Build history of the part. All positions in model axes, mm. Face numbers are marked on the shaded views. Give positions to 0.01 mm unless a question says otherwise; leave off trailing zeros. Order: outer loops, then holes, each group sorted by start corner. A loop starts at its lowest first (then second) coordinate and runs counter-clockwise, first axis right, second up. Notation, with made-up numbers: (15.5, 87.5) -> (62.5, 87.5) arc R23 ccw to (62.5, 96.5) -> close; hole circle Ø3 at (22, 37.5). An arc over 180 degrees is marked (long way). One line per item, written item: value. Start each with the question number.
(1) Saw through at B-B on z = 21.75. Give the cut face in (x, y), plus the area to 4 significant figures.
(2) Saw through at D-D on x = 0. Give the cut face in (y, z), plus the area to 3 significant figures.
(3) Two-plate mould, pull along Y, no slides. Class the marked faces 1, 2, 3 and 4: +Y half, -Y half, draft (parallel to the pull), parting line (faces both ways), or undercut.
(4) Probe line 1 (Y direction, x = 10, z = 2.75); line 2 (Z direction, x = 23, y = 1.25); line 3 (Y direction, x = -2, z = 23.75). List the from-to ranges inside material, lowest first.
(5) Saw through at C-C on y = 1. Give the cut face in (x, z), plus the area to 3 significant figures.
(6) Pin check, flat tips, straight feed: pin 1 (0.5 mm diameter, centred on y = 3.5, z = 9, fed in from -X); pin 2 (2 mm diameter, centred on x = 3, y = 0, fed in from +Z); pin 3 (4 mm diameter, centred on y = 0, z = 19.5, fed in from +X); pin 4 (0.7 mm diameter, centred on x = -26.5, y = -3.5, fed in from +Z). Stop position of each tip, or through.
(7) Saw through at A-A on x = 21.5. Give the cut face in (y, z), plus the area to 3 significant figures.
```python
from build123d import *

# Parameters (mm, degrees)
SKETCH1_W           = 90
SKETCH1_H           = 8
BOSS_EXTRUDE1_DEPTH = 12.6
SKETCH2_W           = 90
SKETCH2_H           = 6.8
CUT_EXTRUDE1_DEPTH  = 12
BOSS_EXTRUDE2_DEPTH = 0.6
CUT_EXTRUDE2_DEPTH  = 9
CUT_EXTRUDE4_DEPTH  = 0.6
CUT_EXTRUDE5_DEPTH  = 0.6
FILLET1_R           = 0.6


with BuildPart() as part:
    # Sketch1 → Boss-Extrude1 (new body)
    with BuildSketch(Plane.XY):
        Rectangle(SKETCH1_W, SKETCH1_H)
    extrude(amount=BOSS_EXTRUDE1_DEPTH)

    # Sketch2 → Cut-Extrude1 (cut)
    with BuildSketch(Plane.XY.offset(12.6)):
        Rectangle(SKETCH2_W, SKETCH2_H)
    extrude(amount=-CUT_EXTRUDE1_DEPTH, mode=Mode.SUBTRACT)

    # Sketch8 → Boss-Extrude2 (add)
    with BuildSketch(Plane.XZ.offset(4)):
        with BuildLine():
            Line((6.4, 25.4), (13.6, 15.8))
            ThreePointArc((13.6, 15.8), (16.422291236, 13.444582472), (20, 12.6))
            Line((20, 12.6), (-20, 12.6))
            ThreePointArc((-20, 12.6), (-16.422291236, 13.444582472), (-13.6, 15.8))
            Line((-13.6, 15.8), (-6.4, 25.4))
            ThreePointArc((-6.4, 25.4), (0, 28.6), (6.4, 25.4))
        make_face()
    extrude(amount=-BOSS_EXTRUDE2_DEPTH)

    # Sketch4 → Cut-Extrude2 (cut, through all)
    with BuildSketch(Plane(origin=(0, 4, 0), x_dir=(1, 0, 0), z_dir=(0, 1, 0))):
        with BuildLine():
            Line((-1.5, -3.1), (-1.5, -32.05439328))
            Line((-1.5, -32.05439328), (1.5, -32.05439328))
            Line((1.5, -32.05439328), (1.5, -3.1))
            ThreePointArc((1.5, -3.1), (0, -1.6), (-1.5, -3.1))
        make_face()
    extrude(amount=-CUT_EXTRUDE2_DEPTH, mode=Mode.SUBTRACT)

    # Sketch6 → Cut-Extrude4 (cut)
    with BuildSketch(Plane(origin=(0, 4, 0), x_dir=(1, 0, 0), z_dir=(0, 1, 0))):
        with BuildLine():
            Line((-42.5, -9.1), (-42.5, -7.1))
            Line((-42.5, -7.1), (-45, -7.1))
            Line((-45, -7.1), (-45, -12.6))
            Line((-45, -12.6), (-39, -12.6))
            ThreePointArc((-39, -12.6), (-41.474873734, -11.574873734), (-42.5, -9.1))
        make_face()
    cut_extrude4 = extrude(amount=-CUT_EXTRUDE4_DEPTH, mode=Mode.SUBTRACT)

    # Mirror1: Cut-Extrude4 across plane
    add(cut_extrude4.mirror(Plane(origin=(0, 0, 0), x_dir=(0, 0, 1), z_dir=(1, 0, 0))), mode=Mode.SUBTRACT)

    # Sketch7 → Cut-Extrude5 (cut)
    with BuildSketch(Plane(origin=(0, 4, 0), x_dir=(1, 0, 0), z_dir=(0, 1, 0))):
        with BuildLine():
            Line((-4.5, -4.6), (-4.5, -6.6))
            ThreePointArc((-4.5, -6.6), (-6, -8.1), (-7.5, -6.6))
            Line((-7.5, -6.6), (-7.5, -4.6))
            ThreePointArc((-7.5, -4.6), (-6, -3.1), (-4.5, -4.6))
        make_face()
    cut_extrude5 = extrude(amount=-CUT_EXTRUDE5_DEPTH, mode=Mode.SUBTRACT)

    # Mirror2: Cut-Extrude5 across plane
    add(cut_extrude5.mirror(Plane(origin=(0, 0, 0), x_dir=(0, 0, 1), z_dir=(1, 0, 0))), mode=Mode.SUBTRACT)

    # Fillet1
    fillet1_edges = [part.edges().sort_by_distance(p)[0] for p in [
        (45, -3.7, 12.6),
        (-45, -3.7, 12.6),
        (-1.5, -3.7, 28.458116823),
        (1.5, -3.7, 28.458116823),
        (1.5, 3.7, 12.6),
        (-1.5, 3.7, 12.6),
        (-45, 3.7, 7.1),
        (45, 3.7, 7.1),
    ]]
    fillet(fillet1_edges, radius=FILLET1_R)


solid = part.part
```
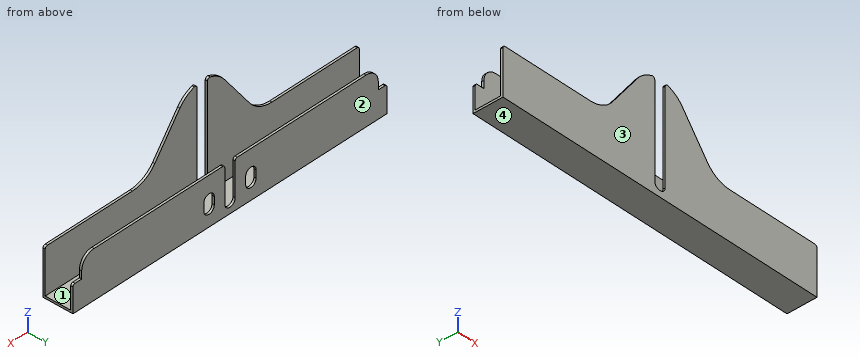
Results below:
1. outline: (-9.14, -4) -> (-1.5, -4) -> (-1.5, -3.4) -> (-9.14, -3.4) -> close; (1.5, -4) -> (9.14, -4) -> (9.14, -3.4) -> (1.5, -3.4) -> close
1. area: 9.165 mm²
2. outline: (-4, 0) -> (4, 0) -> (4, 1.6) -> (3.4, 1.6) -> (3.4, 0.6) -> (-3.4, 0.6) -> (-3.4, 1.6) -> (-4, 1.6) -> close
2. area: 6.00 mm²
3. face 1: undercut
3. face 2: +Y half
3. face 3: -Y half
3. face 4: draft
4. line 1: y = -4 to -3.4, 3.4 to 4
4. line 2: z = 0 to 0.6
4. line 3: y = -4 to -3.4
5. outline: (-45, 0) -> (45, 0) -> (45, 0.6) -> (-45, 0.6) -> close
5. area: 54.0 mm²
6. pin 1: stops at x = -42.5
6. pin 2: stops at z = 0.6
6. pin 3: passes through
6. pin 4: stops at z = 12.6
7. outline: (-4, 0) -> (4, 0) -> (4, 12.6) -> (3.4, 12.6) -> (3.4, 0.6) -> (-3.4, 0.6) -> (-3.4, 12.6) -> (-4, 12.6) -> close
7. area: 19.2 mm²
